```python
from build123d import *

# Parameters (mm, degrees)
SKETCH1_R           = 6.025
SKETCH1_R_2         = 1.585
BOSS_EXTRUDE1_DEPTH = 7.6
CHAMFER1_SIZE       = 0.5
CHAFL_N1_SIZE       = 0.4
CHAFL_N2_SIZE       = 1


with BuildPart() as part:
    # Sketch1 → Boss-Extrude1 (new body)
    with BuildSketch(Plane.XY):
        with Locations(Location((0, 0, 0), (0, 0, 180))):
            Circle(SKETCH1_R)
        with Locations(Location((0, 0, 0), (0, 0, 180))):
            Circle(SKETCH1_R_2, mode=Mode.SUBTRACT)
    extrude(amount=BOSS_EXTRUDE1_DEPTH)

    # Chamfer1
    chamfer1_edges = [part.edges().sort_by_distance(p)[0] for p in [
        (6.025, 0, 0),
        (6.025, 0, 7.6),
    ]]
    chamfer(chamfer1_edges, length=CHAMFER1_SIZE)

    # Chaflán1
    chafl_n1_edges = [part.edges().sort_by_distance(p)[0] for p in [
        (1.585, 0, 7.6),
    ]]
    chamfer(chafl_n1_edges, length=CHAFL_N1_SIZE)

    # Chaflán2
    chafl_n2_edges = [part.edges().sort_by_distance(p)[0] for p in [
        (1.585, 0, 0),
    ]]
    chamfer(chafl_n2_edges, length=CHAFL_N2_SIZE)


solid = part.part
```
For this review, take the finished solid that the model builds, in its own axes (mm). Coordinates: 2 decimals unless noted, no trailing zeros. Loops run counter-clockwise (first coordinate to the right, second up) from the corner with the lowest first, then second, coordinate; pieces in that order, holes last.
1. For line 1 (Y direction, x = 0, z = 4.5) (3 decimals); line 2 (X direction, y = 1.25, z = 4.75); line 3 (Y direction, x = -0.5, z = 5), list the stretches that pass through material, from the lowest coordinate up.
2. Add section A-A, the plane y = 0. Give the boundary of the cut face in (x, z) (3 decimals), then the cut area to 3 significant figures.
3. Mouldability with a two-part tool opening along X and no side actions: class faces 1 (the flat face through (3, 1, 0)), 2 (the cylindrical face through (0.34, 1.55, 4.06)), 3 (the cylindrical face through (4.44, -4.07, 3.75)) as +X half, -X half, draft (parallel to the pull), parting line (faces both ways), or undercut.
4. Add section C-C, the plane z = 4. Give the boundary of the cut face in (x, y) (3 decimals).
Result:
1. line 1: y = -6.025 to -1.585, 1.585 to 6.025
1. line 2: x = -5.89 to -0.97, 0.97 to 5.89
1. line 3: y = -6 to -1.5, 1.5 to 6
2. outline: (-6.025, 0.5) - (-5.525, 0) - (-2.585, 0) - (-1.585, 1) - (-1.585, 7.2) - (-1.985, 7.6) - (-5.525, 7.6) - (-6.025, 7.1) - close; (1.585, 1) - (2.585, 0) - (5.525, 0) - (6.025, 0.5) - (6.025, 7.1) - (5.525, 7.6) - (1.985, 7.6) - (1.585, 7.2) - close
2. area: 65.8 mm2
3. face 1: draft
3. face 2: undercut
3. face 3: parting line
4. outline: circle Ø12.05 at (0, 0); hole circle Ø3.17 at (0, 0)
